CAD build for the part. Positions are in the model's coordinates, mm. Face numbers are marked on the shaded views. A direction names the side the tool comes from. Coordinates: 2 decimals unless noted, no trailing zeros. Loops run counter-clockwise (first coordinate to the right, second up) from the corner with the lowest first, then second, coordinate; pieces in that order, holes last. Notation, with made-up numbers: (-22, -12) -> (-14, -12) arc R33 cw to (-14, 20) -> close; hole circle Ø1 at (11, -26.5). An arc over 180 degrees is marked (long way). Write each question's results on one line, items separated by ' | '.
```python
from build123d import *

# Parameters (mm, degrees)
SKETCH1_W            = 24.892
SKETCH1_H            = 17.78
BOSS_EXTRUDE1_DEPTH  = 20.32
SKETCH2_W            = 6.35
SKETCH2_H            = 17.78
BOSS_EXTRUDE2_DEPTH  = 17.78
SKETCH16_W           = 6.35
SKETCH16_H           = 12.7
BOSS_EXTRUDE11_DEPTH = 12.7
SKETCH20_W           = 8.89
SKETCH20_H           = 3.048
BOSS_EXTRUDE12_DEPTH = 39.624
SKETCH21_W           = 8.89
SKETCH21_H           = 7.539530378
BOSS_EXTRUDE13_DEPTH = 3.302
SKETCH22_W           = 6.35
SKETCH22_H           = 7.539530378
BOSS_EXTRUDE14_DEPTH = 12.7
SKETCH18_R           = 2.547686281
SKETCH18_R_2         = 2.439237793
CUT_EXTRUDE11_DEPTH  = 72.056471626
FILLET8_R            = 2.54


with BuildPart() as part:
    # Sketch1 → Boss-Extrude1 (new body)
    with BuildSketch(Plane.XY):
        with Locations((12.446, 8.89)):
            Rectangle(SKETCH1_W, SKETCH1_H)
    extrude(amount=BOSS_EXTRUDE1_DEPTH)

    # Sketch2 → Boss-Extrude2 (add)
    with BuildSketch(Plane(origin=(24.892, 0, 0), x_dir=(0, 0, -1), z_dir=(1, 0, 0))):
        with Locations((-17.145, 8.89)):
            Rectangle(SKETCH2_W, SKETCH2_H)
    extrude(amount=BOSS_EXTRUDE2_DEPTH)

    # Sketch16 → Boss-Extrude11 (add)
    with BuildSketch(Plane(origin=(42.672, 0, 0), x_dir=(0, 0, -1), z_dir=(1, 0, 0))):
        with Locations((-17.145, 11.43)):
            Rectangle(SKETCH16_W, SKETCH16_H)
    extrude(amount=BOSS_EXTRUDE11_DEPTH)

    # Sketch20 → Boss-Extrude12 (add)
    with BuildSketch(Plane.XZ):
        with Locations((38.227, 18.796)):
            Rectangle(SKETCH20_W, SKETCH20_H)
    extrude(amount=BOSS_EXTRUDE12_DEPTH)

    # Sketch21 → Boss-Extrude13 (add)
    with BuildSketch(Plane(origin=(0, 0, 17.272), x_dir=(-1, 0, 0), z_dir=(0, 0, -1))):
        with Locations((-38.227, -35.854234811)):
            Rectangle(SKETCH21_W, SKETCH21_H)
    extrude(amount=BOSS_EXTRUDE13_DEPTH)

    # Sketch22 → Boss-Extrude14 (add)
    with BuildSketch(Plane(origin=(42.672, 0, 0), x_dir=(0, 0, -1), z_dir=(1, 0, 0))):
        with Locations((-17.145, -35.854234811)):
            Rectangle(SKETCH22_W, SKETCH22_H)
    extrude(amount=BOSS_EXTRUDE14_DEPTH)

    # Sketch18 → Cut-Extrude11 (cut, through all)
    with BuildSketch(Plane.XY.offset(20.32)):
        with Locations((49.940213472, 11.366437705)):
            Circle(SKETCH18_R)
        with Locations((49.693177742, -35.877562295)):
            Circle(SKETCH18_R_2)
    extrude(amount=-CUT_EXTRUDE11_DEPTH, mode=Mode.SUBTRACT)

    # Fillet8
    fillet8_edges = [part.edges().sort_by_distance(p)[0] for p in [
        (24.892, 8.89, 13.97),
        (42.672, 5.08, 17.145),
        (55.372, 5.08, 17.145),
        (33.782, 0, 18.796),
        (38.227, 0, 17.272),
        (33.782, -16.042234811, 17.272),
        (38.227, -32.084469622, 17.272),
        (33.782, -32.084469622, 15.621),
        (42.672, -32.084469622, 18.796),
        (55.372, -32.084469622, 17.145),
    ]]
    fillet(fillet8_edges, radius=FILLET8_R)


solid = part.part
```
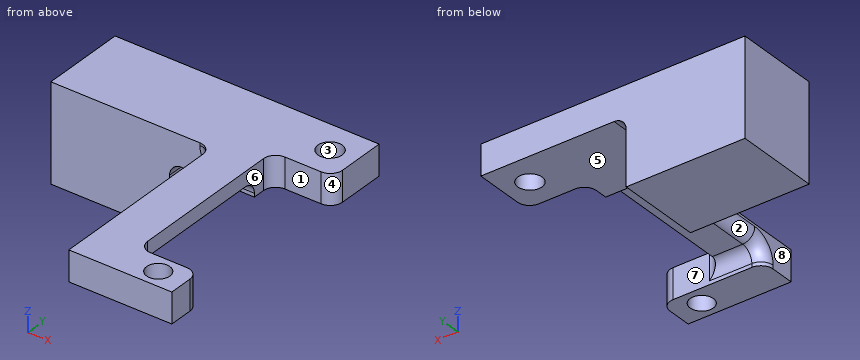
Q1. Cut at A-A on y = -5.5. Write the cut outline in (x, z).
Results are:
outline: (33.78, 19.81) arc R2.54 ccw to (36.32, 17.27) -> (42.67, 17.27) -> (42.67, 20.32) -> (33.78, 20.32) -> close
Q2. Drop flat-ended pins along their axis: pin 1 (1.9 mm diameter, centred on y = -7, z = 18.5, fed in from +X); pin 2 (1.9 mm diameter, centred on x = 40.5, y = -19, fed in from -Z); pin 3 (12 mm diameter, centred on y = -16.5, z = 13.5, fed in from -X). Give the stop position or say it passes through.
Results are:
pin 1: x = 42.67 | pin 2: z = 17.27 | pin 3: x = 33.8
Q3. Cut at C-C on z = 9.75. Write the cut outline in (x, y), and give its area (3 significant figures).
Results are:
outline: (0, 0) -> (24.89, 0) -> (24.89, 17.78) -> (0, 17.78) -> close | area: 443 mm^2
Q4. Wall check: L1, parallel to Y at x = 46, z = 19.75; L2, parallel to Z at x = 39.5, y = 5.5; L3, parallel to X at y = 11.5, z = 9. Give the ranges that are in metal, low to high. Write a range as from..to.
Results are:
L1: -39.62..-32.08, 5.08..17.78 | L2: 13.97..20.32 | L3: 0..24.89
Q5. Pull direction X, two halves, no side cores. Call the marked faces 1, 2, 3 and 4: +X half, -X half, draft (parallel to the pull), parting line (faces both ways), or undercut.
Results are:
face 1: draft | face 2: -X half | face 3: undercut | face 4: +X half
Q6. Cut at B-B on x = 19.5. Write the cut outline in (y, z).
Results are:
outline: (0, 0) -> (17.78, 0) -> (17.78, 20.32) -> (0, 20.32) -> close
Q7. Which spindle directions (+Z, -Z, +X, -X, +Y, -Y) get a long thin tool onto all of the face, cutting with end or side? Do the marked faces 5, 6, 7 and 8. Say none if no direction does.
Results are:
face 5: -Z, +X, +Y, -Y | face 6: +Z, -Z, +X | face 7: -Z, +X | face 8: +Z, -Z, -X, -Y
Q8. Cut at D-D on y = 3.5. Write the cut outline in (x, z).
Results are:
outline: (0, 0) -> (24.89, 0) -> (24.89, 11.43) arc R2.54 cw to (27.43, 13.97) -> (42.86, 13.97) -> (42.86, 20.32) -> (0, 20.32) -> close
